Work out the finished part from the listing and answer in its coordinate system (mm). A direction names the side the tool comes from. Give positions to 0.01 mm unless a question says otherwise; leave off trailing zeros. Loops run counter-clockwise (first coordinate to the right, second up) from the corner with the lowest first, then second, coordinate; pieces in that order, holes last. Notation, with made-up numbers: (25, 40.5) - (38, 40.5) arc R29 cw to (38, 70.5) - close; hole circle Ø8 at (70, -40). An arc over 180 degrees is marked (long way). Use CSV: the item, a comma, the result in double quotes.
from build123d import *

# Parameters (mm, degrees)
BOX007_W                  = 0.4
BOX007_H                  = 1.1
BOX007_DEPTH              = 2.5
BOX005_W                  = 0.4
BOX005_H                  = 1.1
BOX005_DEPTH              = 2.5
BOX006_W                  = 0.4
BOX006_H                  = 1.1
BOX006_DEPTH              = 2.5
BOX008_W                  = 0.4
BOX008_H                  = 1.1
BOX008_DEPTH              = 2.5
BOX004_W                  = 15.7
BOX004_H                  = 12.3
BOX004_DEPTH              = 14.8
BOX009_W                  = 0.4
BOX009_H                  = 1.1
BOX009_DEPTH              = 2.5
FUSION001_PLACEMENT_ANGLE = 90


with BuildPart() as obj1:
    # Box007 → Box007 (new body)
    with BuildSketch(Plane(origin=(3.95, 10.6, -2), x_dir=(1, 0, 0), z_dir=(0, 0, 1))):
        with Locations((0.2, 0.55)):
            Rectangle(BOX007_W, BOX007_H)
    extrude(amount=BOX007_DEPTH)


with BuildPart() as obj2:
    # Box005 → Box005 (new body)
    with BuildSketch(Plane(origin=(1.45, 5.6, -2), x_dir=(1, 0, 0), z_dir=(0, 0, 1))):
        with Locations((0.2, 0.55)):
            Rectangle(BOX005_W, BOX005_H)
    extrude(amount=BOX005_DEPTH)


with BuildPart() as obj3:
    # Box006 → Box006 (new body)
    with BuildSketch(Plane(origin=(14.15, 10.6, -2), x_dir=(1, 0, 0), z_dir=(0, 0, 1))):
        with Locations((0.2, 0.55)):
            Rectangle(BOX006_W, BOX006_H)
    extrude(amount=BOX006_DEPTH)


with BuildPart() as obj4:
    # Box008 → Box008 (new body)
    with BuildSketch(Plane(origin=(14.15, 0.6, -2), x_dir=(1, 0, 0), z_dir=(0, 0, 1))):
        with Locations((0.2, 0.55)):
            Rectangle(BOX008_W, BOX008_H)
    extrude(amount=BOX008_DEPTH)


with BuildPart() as cuerpo:
    # Box004 → Box004 (new body)
    with BuildSketch(Plane.XY.offset(-1)):
        with Locations((7.85, 6.15)):
            Rectangle(BOX004_W, BOX004_H)
    extrude(amount=BOX004_DEPTH)


with BuildPart() as relay:
    # Box009 → Box009 (new body)
    with BuildSketch(Plane(origin=(3.95, 0.6, -2), x_dir=(1, 0, 0), z_dir=(0, 0, 1))):
        with Locations((0.2, 0.55)):
            Rectangle(BOX009_W, BOX009_H)
    extrude(amount=BOX009_DEPTH)

    # Fusion001: union obj1, obj2, obj3, obj4, cuerpo
    add(obj1.part)
    add(obj2.part)
    add(obj3.part)
    add(obj4.part)
    add(cuerpo.part)


with BuildPart() as relay_1:
    # Fusion001 placement: moved
    add(relay.part.moved(Location((12.4, 0, 1.6))).rotate(Axis((12.4, 0, 1.6), (0, 0, 1)), FUSION001_PLACEMENT_ANGLE))


solid = relay_1.part
Item 1: Given P1, Ø3.5, axis at x = 8.5, y = 10.5, coming from the -Z side; P2, Ø0.8, axis at x = 11, z = 0, coming from the -Y side; P3, Ø0.5, axis at x = 6, z = 0, coming from the -Y side, each flat-ended and moving along its own axis, determine where each tip first touches the part or whether it passes through.
Determined:
P1,"stops at z = 0.6"
P2,"stops at y = 3.95"
P3,"stops at y = 1.45"
Item 2: For faces 4 (the flat face through (6, 1.45, 0)), 5 (the flat face through (11, 4.35, 0)), 6 (the flat face through (1, 14.55, 0)), determine the directions among +Z, -Z, +X, -X, +Y, -Y from which every point of the face is accessible in a straight line to the end or side of a thin tool.
Determined:
face 4,"-Z, +X, -X, -Y"
face 5,"-Z, +X, -X"
face 6,"-Z, +X, -X, +Y"
Item 3: Find the intervals of material crossed by line 1 (Z direction, x = 5.25, y = 5.25), in increasing order.
Determined:
line 1,"z = 0.6 to 15.4"
Item 4: A cutting plane is placed at B-B on x = 9.5. Determine the outline of the cut face in (y, z).
Determined:
outline,"(0, 0.6) - (15.7, 0.6) - (15.7, 15.4) - (0, 15.4) - close"
Item 5: A cutting plane is placed at A-A on y = 12.75. Determine the outline of the cut face in (x, z).
Determined:
outline,"(0.1, 0.6) - (12.4, 0.6) - (12.4, 15.4) - (0.1, 15.4) - close"
Item 6: The mould has two halves that part along Y. Classify faces 1 (the flat face through (12.4, 8, 8)), 2 (the flat face through (6, 1.85, 0)), 3 (the flat face through (1, 4.35, 0)): pulls with the +Y half, pulls with the -Y half, needs draft (parallel to the pull), parting line crosses it, or undercut.
Determined:
face 1,"needs draft"
face 2,"pulls with the +Y half"
face 3,"undercut"
